```python
from build123d import *

# Parameters (mm, degrees)
SKETCH_1_R          = 2.05
EXTRUDE_1_DEPTH     = 5.95
SKETCH_2_R          = 5
SKETCH_2_R_2        = 4.3
CUT_EXTRUDE_1_DEPTH = 3
FILLET_1_R          = 1
CHAMFER_2_SIZE      = 1
CHAMFER_3_SIZE      = 1
CHAMFER_3_SIZE2     = 0.709809686


with BuildPart() as part:
    # 스케치1 → 보스-돌출1 (new, symmetric)
    with BuildSketch(Plane.XY):
        with BuildLine():
            Line((-9.3, -4), (-9.3, -5.916283943))
            Line((-9.3, -5.916283943), (-12, -3.906505398))
            Line((-12, -3.906505398), (-12, 4.145721859))
            Line((-12, 4.145721859), (-12, 7.645721859))
            Line((-12, 7.645721859), (-8.7, 3.712694326))
            Line((-8.7, 3.712694326), (7, 3.712694326))
            Line((7, 3.712694326), (8, 6))
            Line((8, 6), (16, 6))
            Line((16, 6), (17, 3.712694326))
            Line((17, 3.712694326), (20, 3.712694326))
            Line((20, 3.712694326), (24.97481487, 3.712694326))
            Line((24.97481487, 3.712694326), (24.97481487, -4.364515181))
            ThreePointArc((24.97481487, -4.364515181), (27.06415919, -4.568973756), (29.05933214, -5.222003534))
            ThreePointArc((29.05933214, -5.222003534), (30.020110844, -7.978170358), (27.746673373, -9.808753146))
            Line((27.746673373, -9.808753146), (21.488254287, -11.89950036))
            Line((21.488254287, -11.89950036), (19.357468482, -2.858721645))
            Line((19.357468482, -2.858721645), (14.656995804, -4))
            Line((14.656995804, -4), (13.992506615, -4))
            Line((13.992506615, -4), (-9.3, -4))
        make_face()
        Circle(SKETCH_1_R, mode=Mode.SUBTRACT)
    extrude(amount=EXTRUDE_1_DEPTH, both=True)

    # 스케치2 → 컷-돌출1 (cut)
    with BuildSketch(Plane.XZ.offset(4)):
        with Locations(Location((13, 0, 0), (0, 0, 270))):
            Circle(SKETCH_2_R)
        with Locations(Location((13, 0, 0), (0, 0, 270))):
            Circle(SKETCH_2_R_2, mode=Mode.SUBTRACT)
    extrude(amount=-CUT_EXTRUDE_1_DEPTH, mode=Mode.SUBTRACT)

    # 필렛1
    # the kernel refuses this fillet: 1 mm, written as the material it takes off along each edge
    with BuildSketch(Plane(origin=(13, -4, 0), x_dir=(0.9752421696657375, 0, -0.22113957245519109), z_dir=(-0.22113957245519109, 0, -0.9752421696657375))) as fillet_1_piece_1:
        with BuildLine():
            CenterArc((4.3 - FILLET_1_R, -FILLET_1_R), FILLET_1_R, 0, 90)
            Line((4.3 - FILLET_1_R, 0), (4.3 - FILLET_1_R, FILLET_1_R * 0.02))
            Line((4.3 - FILLET_1_R, FILLET_1_R * 0.02), (4.3 + FILLET_1_R * 0.02, FILLET_1_R * 0.02))
            Line((4.3 + FILLET_1_R * 0.02, FILLET_1_R * 0.02), (4.3 + FILLET_1_R * 0.02, -FILLET_1_R))
            Line((4.3 + FILLET_1_R * 0.02, -FILLET_1_R), (4.3, -FILLET_1_R))
        make_face()
    revolve(axis=Axis((13, -4, 0), (0, -1, 0)), revolution_arc=282.775974377, mode=Mode.SUBTRACT)
    with BuildSketch(Plane(origin=(13, -4, 0), x_dir=(0, 0, -1), z_dir=(-1, 0, 0))) as fillet_1_piece_2:
        with BuildLine():
            CenterArc((4.3 - FILLET_1_R, -FILLET_1_R), FILLET_1_R, 0, 90)
            Line((4.3 - FILLET_1_R, 0), (4.3 - FILLET_1_R, FILLET_1_R * 0.02))
            Line((4.3 - FILLET_1_R, FILLET_1_R * 0.02), (4.3 + FILLET_1_R * 0.02, FILLET_1_R * 0.02))
            Line((4.3 + FILLET_1_R * 0.02, FILLET_1_R * 0.02), (4.3 + FILLET_1_R * 0.02, -FILLET_1_R))
            Line((4.3 + FILLET_1_R * 0.02, -FILLET_1_R), (4.3, -FILLET_1_R))
        make_face()
    revolve(axis=Axis((13, -4, 0), (0, -1, 0)), revolution_arc=102.614973236, mode=Mode.SUBTRACT)

    # 모따기2
    chamfer_2_edges = [part.edges().sort_by_distance(p)[0] for p in [
        (24.97481487, -0.325910428, -5.95),
        (24.97481487, -0.325910428, 5.95),
    ]]
    chamfer(chamfer_2_edges, length=CHAMFER_2_SIZE)

    # 모따기3
    chamfer_3_edges = [part.edges().sort_by_distance(p)[0] for p in [
        (-12, 7.645721859, 0),
    ]]
    chamfer_3_side = [part.faces().sort_by_distance(p)[0] for p in [
        (-10.35, 5.679208093, 0),
    ]]
    chamfer(chamfer_3_edges, length=CHAMFER_3_SIZE, length2=CHAMFER_3_SIZE2, reference=chamfer_3_side[0])


solid = part.part
```
Could you check a few things on this model? Use its own coordinates, in mm. A direction names the side the tool comes from. Coordinates: 2 decimals unless noted, no trailing zeros. Write each loop counter-clockwise with the first axis right and the second up, starting at its lowest first coordinate (ties: lowest second). Pieces come first, ordered by that corner, then holes. Notation, with made-up numbers: (-18, -2) - (25, -2) arc R16 cw to (25, 27) - close; hole circle Ø6 at (-33.5, 33.5). An arc over 180 degrees is marked (long way). Use a Markdown table: item, result.
Q1. Which directions (+Z, -Z, +X, -X, +Y, -Y) give clear straight access to the entire face, cutting with the end or side of a thin tool? Please do faces 1 (the flat face through (7.493, 4.84, 0.083)), 2 (the cylindrical face through (11.35, -2.01, -3.97)), 3 (the flat face through (13, -4, 0)), 4 (the flat face through (12, 6, 0)).
Geometry check:
| item | result |
|---|---|
| face 1 | +Z, -Z, +Y |
| face 2 | -Y |
| face 3 | +Z, -Z, -Y |
| face 4 | +Z, -Z, +X, +Y |
Q2. Imagine slicing it at C-C (x = 13). List the corners of the cut face in (y, z) for me.
Geometry check:
| item | result |
|---|---|
| outline | (-4, -5.95) - (6, -5.95) - (6, 5.95) - (-4, 5.95) - (-4, 5) - (-1, 5) - (-1, 4.3) - (-3, 4.3) arc R1 ccw to (-4, 3.3) - (-4, -3.3) arc R1 ccw to (-3, -4.3) - (-1, -4.3) - (-1, -5) - (-4, -5) - close |
Q3. Thinking about a two-plate mould opening in Z: for faces 5 (the flat face through (18.61, -3.04, 0.08)), 6 (the flat face through (17, -1, -2)), 7 (the flat face through (24.482, -0.301, 5.443)), which applies, +Z half, -Z half, draft (parallel to the pull), parting line (faces both ways), or undercut?
Geometry check:
| item | result |
|---|---|
| face 5 | draft |
| face 6 | undercut |
| face 7 | +Z half |
Q4. I'm going to push flat-ended pins straight in: pin 1 Ø6 at (x, z) = (1.5, -2.5) entering from +Y; pin 2 Ø3.5 at (x, y) = (0, 0) entering from -Z; pin 3 Ø2.5 at (x, z) = (14, -1.5) entering from +Y; pin 4 Ø3 at (x, z) = (14, 1.5) entering from -Y. Where does each tip first touch, or does it pass through?
Geometry check:
| item | result |
|---|---|
| pin 1 | stops at y = 3.71 |
| pin 2 | passes through |
| pin 3 | stops at y = 6 |
| pin 4 | stops at y = -4 |
Q5. Imagine slicing it at A-A (y = 0). List the corners of the cut face in (x, z) for me, and give its area (3 significant figures).
Geometry check:
| item | result |
|---|---|
| outline | (-12, -5.95) - (-2.05, -5.95) - (-2.05, 5.95) - (-12, 5.95) - close; (2.05, -5.95) - (23.97, -5.95) - (24.97, -4.95) - (24.97, 4.95) - (23.97, 5.95) - (2.05, 5.95) - close |
| area | 390 mm2 |
Q6. Please list where these lines run through material, in increasing order: L1, parallel to X at y = -2.5, z = 0; L2, parallel to Y at x = 0, z = -1; L3, parallel to Y at x = -1.5, z = -3.75.
Geometry check:
| item | result |
|---|---|
| L1 | x = -12 to 8, 8.7 to 17.3, 18 to 24.97 |
| L2 | y = -4 to -2.05, 2.05 to 3.71 |
| L3 | y = -4 to -1.4, 1.4 to 3.71 |
Q7. Imagine slicing it at D-D (z = 0). List the corners of the cut face in (x, y) for me.
Geometry check:
| item | result |
|---|---|
| outline | (-12, -3.91) - (-9.3, -5.92) - (-9.3, -4) - (8, -4) - (8, -1) - (8.7, -1) - (8.7, -3) arc R1 ccw to (9.7, -4) - (14.66, -4) - (17.23, -3.38) arc R1 ccw to (17.3, -3) - (17.3, -1) - (18, -1) - (18, -3.19) - (19.36, -2.86) - (21.49, -11.9) - (27.75, -9.81) arc R2.53 ccw to (29.06, -5.22) arc R9.62 ccw to (24.97, -4.36) - (24.97, 3.71) - (17, 3.71) - (16, 6) - (8, 6) - (7, 3.71) - (-8.7, 3.71) - (-11.36, 6.88) - (-12, 6.94) - close; hole circle Ø4.1 at (0, 0) |
Q8. Imagine slicing it at B-B (x = 0). List the corners of the cut face in (y, z) for me, and give its area (3 significant figures).
Geometry check:
| item | result |
|---|---|
| outline | (-4, -5.95) - (-2.05, -5.95) - (-2.05, 5.95) - (-4, 5.95) - close; (2.05, -5.95) - (3.71, -5.95) - (3.71, 5.95) - (2.05, 5.95) - close |
| area | 43.0 mm2 |
